Part model, mm, in its own coordinate system. Give positions to 0.01 mm unless a question says otherwise; leave off trailing zeros. Order: outer loops, then holes, each group sorted by start corner. A loop starts at its lowest first (then second) coordinate and runs counter-clockwise, first axis right, second up. Notation, with made-up numbers: (25.25, 51.25) - (35.25, 51.25) arc R16 cw to (35.25, 55.25) - close; hole circle Ø1 at (-16, -33). An arc over 180 degrees is marked (long way). One line per item, written item: value.
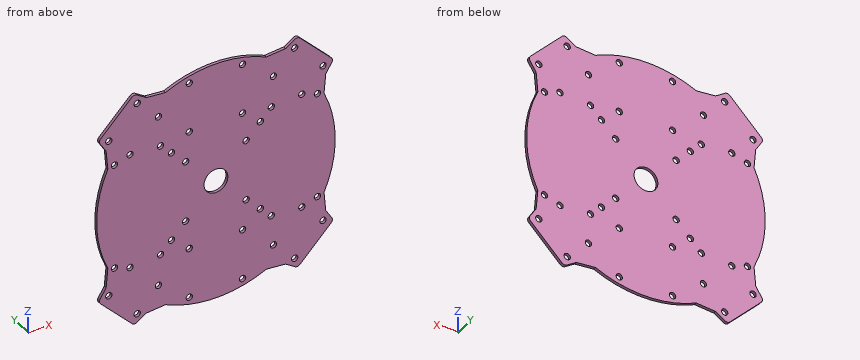
```python
from build123d import *

# Parameters (mm, degrees)
SKETCH_1_R      = 1.6
SKETCH_1_R_2    = 6
EXTRUDE_2_DEPTH = 1.5


with BuildPart() as part:
    # 草图1 → 凸台-拉伸2 (new body)
    with BuildSketch(Plane(origin=(0, 0, 0), x_dir=(1, 0, 0), z_dir=(0, 1, 0))):
        with BuildLine():
            Line((58.010697546, -42.257044027), (42.257044027, -58.010697546))
            ThreePointArc((42.257044027, -58.010697546), (41.057354584, -58.58494555), (39.762791017, -58.279788707))
            Line((39.762791017, -58.279788707), (35.001785669, -55.225039611))
            Line((35.001785669, -55.225039611), (25.377547624, -54.368925652))
            ThreePointArc((25.377547624, -54.368925652), (0, -60), (-25.377547624, -54.368925652))
            Line((-25.377547624, -54.368925652), (-35.001785669, -55.225039611))
            Line((-35.001785669, -55.225039611), (-39.762791017, -58.279788707))
            ThreePointArc((-39.762791017, -58.279788707), (-41.057354584, -58.58494555), (-42.257044027, -58.010697546))
            Line((-42.257044027, -58.010697546), (-58.010697546, -42.257044027))
            ThreePointArc((-58.010697546, -42.257044027), (-58.58494555, -41.057354584), (-58.279788707, -39.762791017))
            Line((-58.279788707, -39.762791017), (-55.225039611, -35.001785669))
            Line((-55.225039611, -35.001785669), (-54.368925652, -25.377547624))
            ThreePointArc((-54.368925652, -25.377547624), (-60, 0), (-54.368925652, 25.377547624))
            Line((-54.368925652, 25.377547624), (-55.225039611, 35.001785669))
            Line((-55.225039611, 35.001785669), (-58.279788707, 39.762791017))
            ThreePointArc((-58.279788707, 39.762791017), (-58.58494555, 41.057354584), (-58.010697546, 42.257044027))
            Line((-58.010697546, 42.257044027), (-42.257044027, 58.010697546))
            ThreePointArc((-42.257044027, 58.010697546), (-41.057354584, 58.58494555), (-39.762791017, 58.279788707))
            Line((-39.762791017, 58.279788707), (-35.001785669, 55.225039611))
            Line((-35.001785669, 55.225039611), (-25.377547624, 54.368925652))
            ThreePointArc((-25.377547624, 54.368925652), (0, 60), (25.377547624, 54.368925652))
            Line((25.377547624, 54.368925652), (35.001785669, 55.225039611))
            Line((35.001785669, 55.225039611), (39.762791017, 58.279788707))
            ThreePointArc((39.762791017, 58.279788707), (41.057354584, 58.58494555), (42.257044027, 58.010697546))
            Line((42.257044027, 58.010697546), (58.010697546, 42.257044027))
            ThreePointArc((58.010697546, 42.257044027), (58.58494555, 41.057354584), (58.279788707, 39.762791017))
            Line((58.279788707, 39.762791017), (55.225039611, 35.001785669))
            Line((55.225039611, 35.001785669), (54.368925652, 25.377547624))
            ThreePointArc((54.368925652, 25.377547624), (60, 0), (54.368925652, -25.377547624))
            Line((54.368925652, -25.377547624), (55.225039611, -35.001785669))
            Line((55.225039611, -35.001785669), (58.279788707, -39.762791017))
            ThreePointArc((58.279788707, -39.762791017), (58.58494555, -41.057354584), (58.010697546, -42.257044027))
        make_face()
        with Locations(Location((39.597979746, 53.881536726, 0), (0, 0, 270))):
            Circle(SKETCH_1_R, mode=Mode.SUBTRACT)
        with Locations(Location((53.881536726, 39.597979746, 0), (0, 0, 270))):
            Circle(SKETCH_1_R, mode=Mode.SUBTRACT)
        with Locations(Location((28.920667351, 43.20422433, 0), (0, 0, 270))):
            Circle(SKETCH_1_R, mode=Mode.SUBTRACT)
        with Locations(Location((43.20422433, 28.920667351, 0), (0, 0, 270))):
            Circle(SKETCH_1_R, mode=Mode.SUBTRACT)
        with Locations(Location((27.860007179, 27.860007179, 0), (0, 0, 270))):
            Circle(SKETCH_1_R, mode=Mode.SUBTRACT)
        with Locations(Location((22.344574285, 22.344574285, 0), (0, 0, 270))):
            Circle(SKETCH_1_R, mode=Mode.SUBTRACT)
        with Locations(Location((15.202795796, 15.202795796, 0), (0, 0, 270))):
            Circle(SKETCH_1_R, mode=Mode.SUBTRACT)
        with Locations(Location((13.4, 54.887976826, 0), (0, 0, 270))):
            Circle(SKETCH_1_R, mode=Mode.SUBTRACT)
        with Locations(Location((13.4, 29.887976826, 0), (0, 0, 270))):
            Circle(SKETCH_1_R, mode=Mode.SUBTRACT)
        with Locations(Location((-13.4, 29.887976826, 0), (0, 0, 270))):
            Circle(SKETCH_1_R, mode=Mode.SUBTRACT)
        with Locations(Location((-13.4, 54.887976826, 0), (0, 0, 270))):
            Circle(SKETCH_1_R, mode=Mode.SUBTRACT)
        with Locations(Location((51.04496003, 26.38323251, 0), (0, 0, 270))):
            Circle(SKETCH_1_R, mode=Mode.SUBTRACT)
        with Locations(Location((-15.202795796, 15.202795796, 0), (0, 0, 270))):
            Circle(SKETCH_1_R, mode=Mode.SUBTRACT)
        with Locations(Location((-22.344574285, 22.344574285, 0), (0, 0, 270))):
            Circle(SKETCH_1_R, mode=Mode.SUBTRACT)
        with Locations(Location((-27.860007179, 27.860007179, 0), (0, 0, 270))):
            Circle(SKETCH_1_R, mode=Mode.SUBTRACT)
        with Locations(Location((-43.20422433, 28.920667351, 0), (0, 0, 270))):
            Circle(SKETCH_1_R, mode=Mode.SUBTRACT)
        with Locations(Location((-51.04496003, 26.38323251, 0), (0, 0, 270))):
            Circle(SKETCH_1_R, mode=Mode.SUBTRACT)
        with Locations(Location((-28.920667351, 43.20422433, 0), (0, 0, 270))):
            Circle(SKETCH_1_R, mode=Mode.SUBTRACT)
        with Locations(Location((-53.881536726, 39.597979746, 0), (0, 0, 270))):
            Circle(SKETCH_1_R, mode=Mode.SUBTRACT)
        with Locations(Location((-39.597979746, 53.881536726, 0), (0, 0, 270))):
            Circle(SKETCH_1_R, mode=Mode.SUBTRACT)
        with Locations(Location((43.20422433, -28.920667351, 0), (0, 0, 270))):
            Circle(SKETCH_1_R, mode=Mode.SUBTRACT)
        with Locations(Location((51.04496003, -26.38323251, 0), (0, 0, 270))):
            Circle(SKETCH_1_R, mode=Mode.SUBTRACT)
        with Locations(Location((53.881536726, -39.597979746, 0), (0, 0, 270))):
            Circle(SKETCH_1_R, mode=Mode.SUBTRACT)
        with Locations(Location((39.597979746, -53.881536726, 0), (0, 0, 270))):
            Circle(SKETCH_1_R, mode=Mode.SUBTRACT)
        with Locations(Location((28.920667351, -43.20422433, 0), (0, 0, 270))):
            Circle(SKETCH_1_R, mode=Mode.SUBTRACT)
        with Locations(Location((27.860007179, -27.860007179, 0), (0, 0, 270))):
            Circle(SKETCH_1_R, mode=Mode.SUBTRACT)
        with Locations(Location((22.344574285, -22.344574285, 0), (0, 0, 270))):
            Circle(SKETCH_1_R, mode=Mode.SUBTRACT)
        with Locations(Location((15.202795796, -15.202795796, 0), (0, 0, 270))):
            Circle(SKETCH_1_R, mode=Mode.SUBTRACT)
        with Locations(Location((13.4, -29.887976826, 0), (0, 0, 270))):
            Circle(SKETCH_1_R, mode=Mode.SUBTRACT)
        with Locations(Location((13.4, -54.887976826, 0), (0, 0, 270))):
            Circle(SKETCH_1_R, mode=Mode.SUBTRACT)
        with Locations(Location((-13.4, -29.887976826, 0), (0, 0, 270))):
            Circle(SKETCH_1_R, mode=Mode.SUBTRACT)
        with Locations(Location((-15.202795796, -15.202795796, 0), (0, 0, 270))):
            Circle(SKETCH_1_R, mode=Mode.SUBTRACT)
        with Locations(Location((-22.344574285, -22.344574285, 0), (0, 0, 270))):
            Circle(SKETCH_1_R, mode=Mode.SUBTRACT)
        with Locations(Location((-27.860007179, -27.860007179, 0), (0, 0, 270))):
            Circle(SKETCH_1_R, mode=Mode.SUBTRACT)
        with Locations(Location((-13.4, -54.887976826, 0), (0, 0, 270))):
            Circle(SKETCH_1_R, mode=Mode.SUBTRACT)
        with Locations(Location((-28.920667351, -43.20422433, 0), (0, 0, 270))):
            Circle(SKETCH_1_R, mode=Mode.SUBTRACT)
        with Locations(Location((-43.20422433, -28.920667351, 0), (0, 0, 270))):
            Circle(SKETCH_1_R, mode=Mode.SUBTRACT)
        with Locations(Location((-51.04496003, -26.38323251, 0), (0, 0, 270))):
            Circle(SKETCH_1_R, mode=Mode.SUBTRACT)
        with Locations(Location((-39.597979746, -53.881536726, 0), (0, 0, 270))):
            Circle(SKETCH_1_R, mode=Mode.SUBTRACT)
        with Locations(Location((-53.881536726, -39.597979746, 0), (0, 0, 270))):
            Circle(SKETCH_1_R, mode=Mode.SUBTRACT)
        with Locations(Location((0, 0, 0), (0, 0, 270))):
            Circle(SKETCH_1_R_2, mode=Mode.SUBTRACT)
    extrude(amount=EXTRUDE_2_DEPTH)


solid = part.part
```
1) Cut at C-C, the plane y = 0.55. Give the number of separate pieces and of enclosed holes in the cut face, then the cut area to 3 significant figures.
Outcome:
separate pieces: 1
enclosed holes: 41
area: 12,300 mm^2
2) Drill centre lines: line 1 along Z through (x, y) = (29.5, 1.2); line 2 along Z through (x, y) = (-42, 1.15); line 3 along Z through (x, y) = (-29, 0.1). Where is each one in solid material? Low to high. Write a range as from..to.
Outcome:
line 1: z = -54.74..-44.7, -41.71..41.71, 44.7..54.74
line 2: z = -58.23..-29.97, -27.87..27.87, 29.97..58.23
line 3: z = -54.69..-44.8, -41.61..-28.98, -26.74..26.74, 28.98..41.61, 44.8..54.69
3) Pin check, flat tip, straight feed: pin 1 (1 mm diameter, centred on x = -1.5, z = -39.5, fed in from -Y). Stop position of the tip, or through.
Outcome:
pin 1: stops at y = 0
4) Cut at A-A, the plane x = 0. Give the cut face in (y, z), then the cut area to 3 significant figures.
Outcome:
outline: (0, -60) - (1.5, -60) - (1.5, -6) - (0, -6) - close; (0, 6) - (1.5, 6) - (1.5, 60) - (0, 60) - close
area: 162 mm^2
5) Cut at B-B, the plane z = 0. Give the cut face in (x, y), then the cut area to 3 significant figures.
Outcome:
outline: (-60, 0) - (-6, 0) - (-6, 1.5) - (-60, 1.5) - close; (6, 0) - (60, 0) - (60, 1.5) - (6, 1.5) - close
area: 162 mm^2
